```python
from build123d import *
from build123d.topology import SkipClean

# Parameters (mm, degrees)
SKETCH_1_R             = 8
EXTRUDE_1_DEPTH        = 55.2
EXTRUDE_2_DEPTH        = 11.8
SKETCH_3_R             = 3
EXTRUDE_3_DEPTH        = 1
SKETCH_4_R             = 2.75
EXTRUDE_4_DEPTH        = 1.6
EXTRUDE_5_DEPTH        = 0.05
EXTRUDE_5_DEPTH_BACK   = 2
SKETCH_5_R             = 8
HOLE_WIZARD_M2_1_D     = 1.6
HOLE_WIZARD_M2_1_DEPTH = 5.2
HOLE_WIZARD_M2_1_TIP   = 0.480688495
SKETCH1_R              = 1.5
EXTRUDE1_DEPTH         = 1.4
CHAMFER_2_SIZE         = 0.1


with BuildPart() as part:
    # 草图1 → 拉伸1 (new body)
    with BuildSketch(Plane.XY):
        with Locations(Location((0, 0, 0), (0, 0, 180))):
            Circle(SKETCH_1_R)
    extrude(amount=EXTRUDE_1_DEPTH)

    # 草图2 → 拉伸2 (add)
    with BuildSketch(Plane(origin=(0, 0, 0), x_dir=(-1, 0, 0), z_dir=(0, 0, -1))):
        with BuildLine():
            Line((-0.748331477, 1.3), (0.748331477, 1.3))
            ThreePointArc((0.748331477, 1.3), (0, -1.5), (-0.748331477, 1.3))
        make_face()
    extrude(amount=EXTRUDE_2_DEPTH)

    # 草图3 → 拉伸3 (add)
    with BuildSketch(Plane(origin=(0, 0, 0), x_dir=(-1, 0, 0), z_dir=(0, 0, -1))):
        with Locations(Location((0, 0, 0), (0, 0, 180))):
            Circle(SKETCH_3_R)
    extrude(amount=EXTRUDE_3_DEPTH)

    # 草图4 → 拉伸4 (add)
    with BuildSketch(Plane(origin=(0, 0, -1), x_dir=(-1, 0, 0), z_dir=(0, 0, -1))):
        Circle(SKETCH_4_R)
    extrude(amount=EXTRUDE_4_DEPTH)

    # 草图5 → 拉伸5 (add, two sides: drawn at the far end of the back side and taken through both)
    with BuildSketch(Plane(origin=(0, 0, 0), x_dir=(-1, 0, 0), z_dir=(0, 0, -1)).offset(-EXTRUDE_5_DEPTH_BACK)):
        Circle(SKETCH_5_R)
    extrude(amount=EXTRUDE_5_DEPTH + EXTRUDE_5_DEPTH_BACK)

    # M2 螺纹孔1
    with Locations(Plane(origin=(5.5, 0, -0.05), x_dir=(-1, 0, 0), z_dir=(0, 0, -1))):
        with Locations((0, 0), (11, 0)):
            Hole(HOLE_WIZARD_M2_1_D / 2, depth=HOLE_WIZARD_M2_1_DEPTH)
            with Locations((0, 0, -(HOLE_WIZARD_M2_1_DEPTH + HOLE_WIZARD_M2_1_TIP / 2))):  # 118° drill point
                Cone(0, HOLE_WIZARD_M2_1_D / 2, HOLE_WIZARD_M2_1_TIP, mode=Mode.SUBTRACT)

    # Sketch1 → Extrude1 (add)
    with SkipClean():  # the faces are left unmerged after this step: merging them gives an invalid solid
        with BuildSketch(Plane(origin=(0, 0, -2.6), x_dir=(-1, 0, 0), z_dir=(0, 0, -1))):
            with Locations(Location((0, 0, 0), (0, 0, 119.926434867))):
                Circle(SKETCH1_R)
        extrude(amount=EXTRUDE1_DEPTH)

    # 倒角2
    chamfer_2_edges = [part.edges().sort_by_distance(p)[0] for p in [
        (0, -1.5, -11.8),
    ]]
    chamfer(chamfer_2_edges, length=CHAMFER_2_SIZE)


solid = part.part
```
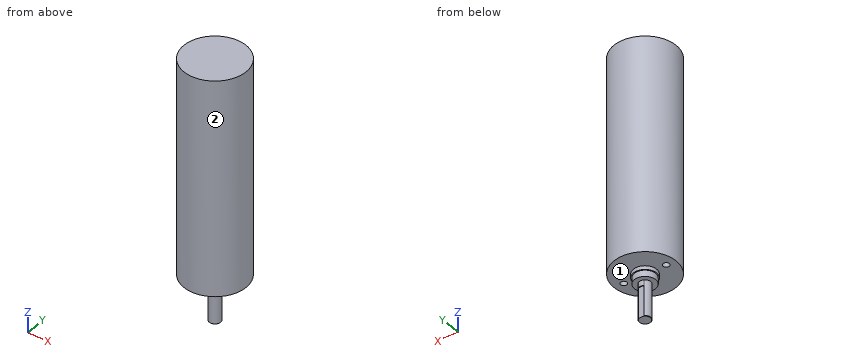
CAD build for the part. Positions are in the model's coordinates, mm. Face numbers are marked on the shaded views. A direction names the side the tool comes from. Coordinates: 2 decimals unless noted, no trailing zeros. Write each loop counter-clockwise with the first axis right and the second up, starting at its lowest first coordinate (ties: lowest second). Pieces come first, ordered by that corner, then holes.
(1) Cut at A-A, the plane z = 3. List the corners of the cut face in (x, y).
(2) Cut at C-C, the plane y = -5. List the corners of the cut face in (x, z) (3 decimals), and give its area (3 significant figures).
(3) 3-axis set-ups, long thin cutter, end or side, ignore diameter. For the marked faces 1 and 2: which of +Z, -Z, +X, -X, +Y, -Y reach the whole face in a straight line?
(4) Drill centre lines: probe 1 along X at (y, z) = (0, 2.9); probe 2 along Z at (x, y) = (-3.5, 3); probe 3 along Y at (x, z) = (-5.5, 2.55). Where is each one in solid material? Low to high.
(5) Flat gauge pins, fed straight in: pin 1 (2 mm diameter, centred on x = -2.5, y = -3, fed in from -Z); pin 2 (3 mm diameter, centred on x = 4, z = -2, fed in from -Y); pin 3 (4 mm diameter, centred on y = -5, z = 33, fed in from -X). Where does each tip first touch, or does it go through?
(6) Cut at B-B, the plane z = 36.5. List the corners of the cut face in (x, y).
Geometry says:
1. outline: circle Ø16 at (0, 0); hole circle Ø1.6 at (-5.5, 0); hole circle Ø1.6 at (5.5, 0)
2. outline: (-6.245, -0.05) - (6.245, -0.05) - (6.245, 55.2) - (-6.245, 55.2) - close
2. area: 690 mm2
3. face 1: -Z
3. face 2: +Z, -Z
4. probe 1: x = -8 to -6.3, -4.7 to 4.7, 6.3 to 8
4. probe 2: z = -0.05 to 55.2
4. probe 3: y = -5.81 to -0.8, 0.8 to 5.81
5. pin 1: stops at z = -1
5. pin 2: stops at y = -1.15
5. pin 3: stops at x = -7.42
6. outline: circle Ø16 at (0, 0)
